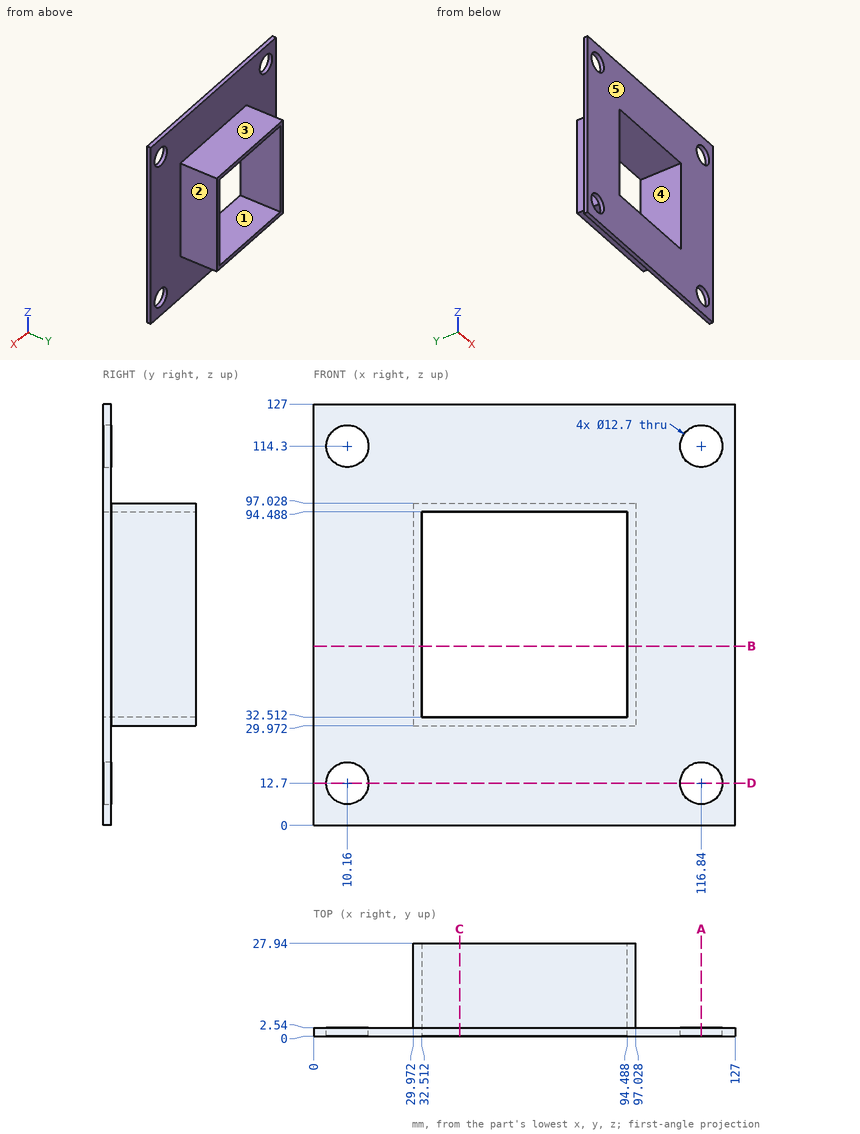
Print and shaded views of the part. All mm, measured from the part's lowest x, y and z. A direction names the side the tool comes from. Round coordinates to 2 decimals unless told otherwise and drop trailing zeros. Write each loop counter-clockwise with the first axis right and the second up, starting at its lowest first coordinate (ties: lowest second). Pieces come first, ordered by that corner, then holes.
Item 1: Cut at B-B, the plane z = 54. Give the cut face in (x, y), plus the area to 3 significant figures.
Results:
outline: (0, 0) - (32.51, 0) - (32.51, 27.94) - (29.97, 27.94) - (29.97, 2.54) - (0, 2.54) - close; (94.49, 0) - (127, 0) - (127, 2.54) - (97.03, 2.54) - (97.03, 27.94) - (94.49, 27.94) - close
area: 294 mm2
Item 2: Cut at A-A, the plane x = 116.84. Give the cut face in (y, z), plus the area to 3 significant figures.
Results:
outline: (0, 0) - (2.54, 0) - (2.54, 6.35) - (0, 6.35) - close; (0, 19.05) - (2.54, 19.05) - (2.54, 107.95) - (0, 107.95) - close; (0, 120.65) - (2.54, 120.65) - (2.54, 127) - (0, 127) - close
area: 258 mm2
Item 3: Cut at D-D, the plane z = 12.7. Give the cut face in (x, y), plus the area to 3 significant figures.
Results:
outline: (0, 0) - (3.81, 0) - (3.81, 2.54) - (0, 2.54) - close; (16.51, 0) - (110.49, 0) - (110.49, 2.54) - (16.51, 2.54) - close; (123.19, 0) - (127, 0) - (127, 2.54) - (123.19, 2.54) - close
area: 258 mm2
Item 4: Cut at C-C, the plane x = 44. Give the cut face in (y, z), plus the area to 3 significant figures.
Results:
outline: (0, 0) - (2.54, 0) - (2.54, 29.97) - (27.94, 29.97) - (27.94, 32.51) - (0, 32.51) - close; (0, 94.49) - (27.94, 94.49) - (27.94, 97.03) - (2.54, 97.03) - (2.54, 127) - (0, 127) - close
area: 294 mm2
Item 5: Probe L1, parallel to X at y = 1.85, z = 114.3; L2, parallel to Z at x = 67, y = 9.25; L3, parallel to Y at x = 98, z = 59.5. List the from-to ranges inside material, lowest first.
Results:
L1: x = 0 to 3.81, 16.51 to 110.49, 123.19 to 127
L2: z = 29.97 to 32.51, 94.49 to 97.03
L3: y = 0 to 2.54
Item 6: Drop flat-ended pins along their axis: pin 1 Ø2 at (y, z) = (12, 99) entering from -X; pin 2 Ø12.5 at (x, y) = (73, 10.5) entering from +Z; pin 3 Ø14 at (y, z) = (21, 64.5) entering from -X; pin 4 Ø8 at (x, y) = (69.5, 16) entering from -Z. Give the stop position or say it passes through.
Results:
pin 1: passes through
pin 2: stops at z = 97.03
pin 3: stops at x = 29.97
pin 4: stops at z = 29.97
Item 7: Which spindle directions (+Z, -Z, +X, -X, +Y, -Y) get a long thin tool onto all of the face, cutting with end or side? Do the marked faces 4 and 5. Say none if no direction does.
Results:
face 4: +Y, -Y
face 5: +Z, -Z, +X, -X, -Y
Item 8: Two-plate mould, pull along Z, no slides. Class the marked faces 1, 2 and 3: +Z half, -Z half, draft (parallel to the pull), parting line (faces both ways), or undercut.
Results:
face 1: undercut
face 2: draft
face 3: +Z half
